Drawing for the job (mm, zero at the part's lowest x, y, z). A direction names the side the tool comes from. Round coordinates to 2 decimals unless told otherwise and drop trailing zeros. Write each loop counter-clockwise with the first axis right and the second up, starting at its lowest first coordinate (ties: lowest second). Pieces come first, ordered by that corner, then holes.
Item 1: Mould opens along Y. For the marked faces 1, 2 and 3 say: +Y half, -Y half, draft (parallel to the pull), parting line (faces both ways), or undercut.
Item 2: Band-saw the part on A-A, the plane x = 21.25. Write the cut outline in (y, z), then the cut area to 3 significant figures.
Item 3: Band-saw the part on C-C, the plane z = 7. Write the cut outline in (x, y), then the cut area to 3 significant figures.
Item 4: Band-saw the part on D-D, the plane x = 36.25. Write the cut outline in (y, z).
Item 5: Drop flat-ended pins along their axis: pin 1 Ø1.8 at (x, y) = (36.25, 21.25) entering from +Z; pin 2 Ø6.5 at (x, y) = (21.5, 36.5) entering from -Z; pin 3 Ø4 at (x, z) = (22.5, 7.5) entering from -Y; pin 4 Ø3 at (y, z) = (14, 9.5) entering from +X. Give the stop position or say it passes through.
Item 6: 3-axis set-ups, long thin cutter, end or side, ignore diameter. For the marked faces 4 and 5: which of +Z, -Z, +X, -X, +Y, -Y reach the whole face in a straight line?
Item 7: Wall check: probe 1 along Y at (x, z) = (21.25, 18); probe 2 along Y at (x, z) = (21.25, 3.85); probe 3 along X at (y, z) = (21, 16). Give the ranges that are in metal, low to high.
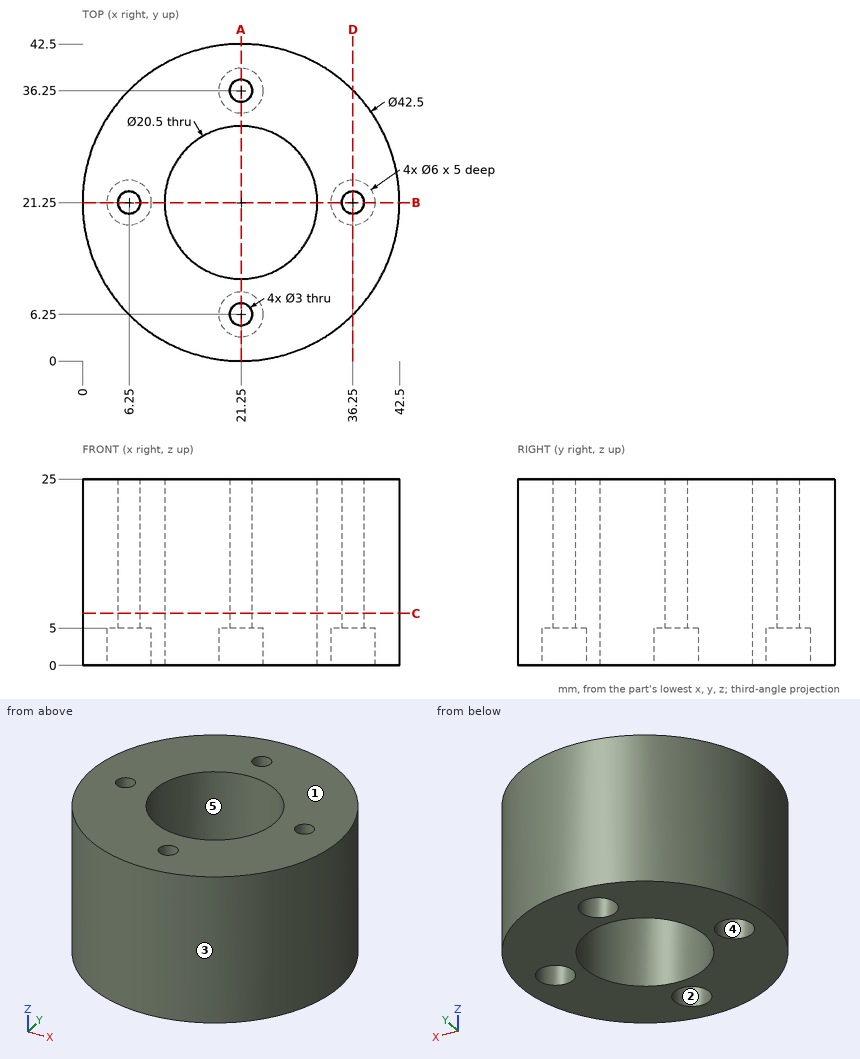
Results:
1. face 1: draft
1. face 2: undercut
1. face 3: parting line
2. outline: (0, 0) - (3.25, 0) - (3.25, 5) - (4.75, 5) - (4.75, 25) - (0, 25) - close; (7.75, 5) - (9.25, 5) - (9.25, 0) - (11, 0) - (11, 25) - (7.75, 25) - close; (31.5, 0) - (33.25, 0) - (33.25, 5) - (34.75, 5) - (34.75, 25) - (31.5, 25) - close; (37.75, 5) - (39.25, 5) - (39.25, 0) - (42.5, 0) - (42.5, 25) - (37.75, 25) - close
2. area: 370 mm2
3. outline: circle Ø42.5 at (21.25, 21.25); hole circle Ø3 at (6.25, 21.25); hole circle Ø20.5 at (21.25, 21.25); hole circle Ø3 at (21.25, 6.25); hole circle Ø3 at (21.25, 36.25); hole circle Ø3 at (36.25, 21.25)
3. area: 1,060 mm2
4. outline: (6.2, 0) - (18.25, 0) - (18.25, 5) - (19.75, 5) - (19.75, 25) - (6.2, 25) - close; (22.75, 5) - (24.25, 5) - (24.25, 0) - (36.3, 0) - (36.3, 25) - (22.75, 25) - close
5. pin 1: passes through
5. pin 2: stops at z = 0
5. pin 3: stops at y = 0
5. pin 4: stops at x = 41.71
6. face 4: -Z
6. face 5: +Z, -Z
7. probe 1: y = 0 to 4.75, 7.75 to 11, 31.5 to 34.75, 37.75 to 42.5
7. probe 2: y = 0 to 3.25, 9.25 to 11, 31.5 to 33.25, 39.25 to 42.5
7. probe 3: x = 0 to 4.77, 7.73 to 11, 31.5 to 34.77, 37.73 to 42.5
